Autodesk Inventor part; units mm, degrees
ref_plane "YZ Plane" through (0, 0, 0) normal (1, 0, 0) x (0, 1, 0)
ref_plane "XZ Plane" through (0, 0, 0) normal (0, 1, 0) x (-1, 0, 0)
ref_plane "XY Plane" through (0, 0, 0) normal (0, 0, 1) x (1, 0, 0)
sketch "Esquisse1" plane through (0, 0, 0) normal (1, 0, 0) x (0, 1, 0)
  line L0 (37, -9) -> (37, 0) construction
  line L1 (0, 7.5) -> (6, 7.5)
  line L2 (12.5, 7) -> (12.5, 0)
  line L3 (0, 7.5) -> (0, -9)
  line L4 (0, 31.5501) -> (0, -31.5501)
  line L5 (37, -4.5) -> (0, -4.5) construction
  line L6 (12.5, 0) -> (39, 0)
  line L7 (39, 0) -> (39, -1.75)
  line L8 (39, -1.75) -> (37, -1.75)
  line L9 (37, -1.75) -> (37, -7.25)
  line L10 (0, -9) -> (39, -9)
  line L11 (39, -9) -> (39, -7.25)
  line L12 (39, -7.25) -> (37, -7.25)
  line L13 (12.5, 7) -> (6, 7)
  line L14 (6, 7) -> (6, 7.5)
  point P0 (0, 0)
  point P1 (6, 7.25)
  dimension "d1" = 9
  dimension "d4" = 0
  dimension "d5" = 74
  dimension "d6" = 25
  dimension "d20" = 2
  dimension "d21" = 2.75
  dimension "d31" = 16.5
  dimension "d32" = 6
  dimension "d33" = 0.5
revolve "Révolution1" add sketch "Esquisse1" angle 360 about axis through (0, 0, 31.5501) along (0, 0, -1)
sketch "Esquisse2" plane through (0, 0, 0) normal (0, 1, 0) x (-1, 0, 0)
  circle A0 centre (0, 4) radius 1.75
  line L0 (-12.5, 7) -> (12.5, 7)
  point P0 (0, 0)
  dimension "d11" = 3.5
  dimension "d12" = 3
extrude "Extrusion1" cut sketch "Esquisse2" along normal through all
sketch "Esquisse3" plane through (0, 0, 7) normal (0, 0, 1) x (1, 0, 0)
  line L0 (-2.75, 8.2) -> (2.75, 8.2)
  line L1 (2.75, 8.2) -> (2.75, 5.8)
  line L2 (2.75, 5.8) -> (-2.75, 5.8)
  line L3 (-2.75, 5.8) -> (-2.75, 8.2)
  line L4 (-2.75, 8.2) -> (2.75, 5.8) construction
  line L5 (2.75, 8.2) -> (-2.75, 5.8) construction
  line L6 (0, 7) -> (0, 0) construction
  point P0 (0, 0)
  dimension "d15" = 5.5
  dimension "d16" = 2.4
  dimension "d17" = 7
extrude "Extrusion2" cut sketch "Esquisse3" against normal blind 6
chamfer "Chanfrein1" distance 3 angle 45 1 edges at (0, -12.5, 0)
sketch "Esquisse4" plane through (0, 0, 7.5) normal (0, 0, 1) x (1, 0, 0)
  arc A0 (-2.5807, 3.25) -> (2.5807, 3.25) centre (0, 0) ccw
  line L0 (-2.5807, 3.25) -> (2.5807, 3.25)
  point P0 (0, 0)
  dimension "d27" = 8.3
  dimension "d28" = 3.25
extrude "Extrusion3" cut sketch "Esquisse4" against normal through all
properties part number "roue"
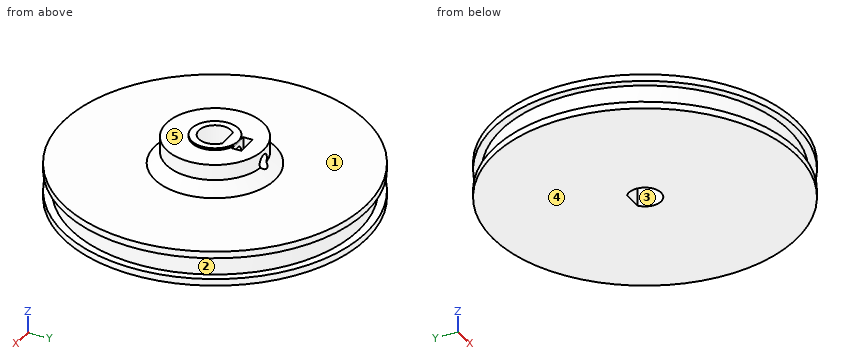
Geometry check sheet. Reference: the model listing, model coordinates, mm. Face numbers are marked on the shaded views. A direction names the side the tool comes from. Round coordinates to 2 decimals unless told otherwise and drop trailing zeros. Order: outer loops, then holes, each group sorted by start corner. A loop starts at its lowest first (then second) coordinate and runs counter-clockwise, first axis right, second up. Notation, with made-up numbers: M 83.5,46.25 L 124.5,46.25 A20 cw 124.5,68.25 Z; hole C -21.5,76 d8. An arc over 180 degrees is marked long. Answer in a Markdown table with one row per item. Add a question column.
Item 1: Draft check along X on the marked faces 1, 2 and 3. Enter one of: released by +X, released by -X, zero draft, split by the parting line, or undercut.
Item 2: Set-up check for the marked faces 4 and 5: record each of +Z, -Z, +X, -X, +Y, -Y from which the full face is reachable in a straight line by a thin tool's end or side.
Item 3: Sectioned sample at C-C, the plane x = -21. Enter the section's corners in (y, z).
Item 4: Material ranges on L1, parallel to X at y = 11.4, z = 4; L2, parallel to X at y = 9.2, z = 4; L3, parallel to Z at x = -21, y = 5, recorded low to high. Write a range as [from, to].
Item 5: Sectioned sample at B-B, the plane z = 4. Enter the section's corners in (x, y).
Item 6: Sectioned sample at D-D, the plane y = -30. Enter the section's corners in (x, z), plus the area to 3 significant figures.
Item 7: Sectioned sample at A-A, the plane y = 0. Enter the section's corners in (x, z).
Item 8: Depth check by flat-ended pin: pin 1 Ø6 at (y, z) = (-11, -5) entering from +X; pin 2 Ø2 at (x, y) = (-20, -1) entering from +Z; pin 3 Ø5.5 at (x, z) = (0, 4) entering from +Y. Enter the tip coordinate at first touch or a pass-through.
Filled in:
| question | item | result |
|---|---|---|
| 1 | face 1 | zero draft |
| 1 | face 2 | split by the parting line |
| 1 | face 3 | undercut |
| 2 | face 4 | -Z, +X, -X, +Y, -Y |
| 2 | face 5 | +Z |
| 3 | outline | M -32.86,-9 L 32.86,-9 L 32.86,-7.25 L 30.46,-7.25 L 30.46,-1.75 L 32.86,-1.75 L 32.86,0 L -32.86,0 L -32.86,-1.75 L -30.46,-1.75 L -30.46,-7.25 L -32.86,-7.25 Z |
| 4 | L1 | x = [-5.13, -1.75], [1.75, 5.13] |
| 4 | L2 | x = [-8.46, -1.75], [1.75, 8.46] |
| 4 | L3 | z = [-9, 0] |
| 5 | outline | M -2.75,5.8 L -2.75,8.2 L -1.75,8.2 L -1.75,12.38 A12.5 ccw long 1.75,12.38 L 1.75,8.2 L 2.75,8.2 L 2.75,5.8 L 1.75,5.8 L 1.75,3.25 L 2.58,3.25 A4.15 cw long -2.58,3.25 L -1.75,3.25 L -1.75,5.8 Z |
| 6 | outline | M -24.92,-9 L 24.92,-9 L 24.92,-7.25 L 21.66,-7.25 L 21.66,-1.75 L 24.92,-1.75 L 24.92,0 L -24.92,0 L -24.92,-1.75 L -21.66,-1.75 L -21.66,-7.25 L -24.92,-7.25 Z |
| 6 | area | 413 mm² |
| 7 | outline | M -39,-9 L -4.15,-9 L -4.15,7.5 L -6,7.5 L -6,7 L -12.5,7 L -12.5,3 L -15.5,0 L -39,0 L -39,-1.75 L -37,-1.75 L -37,-7.25 L -39,-7.25 Z; M 4.15,-9 L 39,-9 L 39,-7.25 L 37,-7.25 L 37,-1.75 L 39,-1.75 L 39,0 L 15.5,0 L 12.5,3 L 12.5,7 L 6,7 L 6,7.5 L 4.15,7.5 Z |
| 8 | pin 1 | stops at x = 37.94 |
| 8 | pin 2 | stops at z = 0 |
| 8 | pin 3 | stops at y = 14.25 |
